Build history of the part. All positions in model axes, mm. A direction names the side the tool comes from. Coordinates: 2 decimals unless noted, no trailing zeros. Loops run counter-clockwise (first coordinate to the right, second up) from the corner with the lowest first, then second, coordinate; pieces in that order, holes last. Notation, with made-up numbers: (80, -6) - (100, -6) arc R29 cw to (100, 16) - close; hole circle Ø6 at (50, 14). An arc over 180 degrees is marked (long way). One line per item, written item: value.
```python
from build123d import *

# Parameters (mm, degrees)
F0_W      = 87.5036269426
F0_H      = 33.1910848618
F1_DEPTH  = 25.4
F1_FACE_W = 87.5036269426
F1_FACE_H = 33.1910848618
F2_DEPTH  = 9.3165077269
F2_TAPER  = -3


with BuildPart() as f1:
    # F0 (on Front) → F1 (new body)
    with BuildSketch(Plane.XZ):
        Rectangle(F0_W, F0_H)
    extrude(amount=F1_DEPTH)

    # F1_face (on face) → F2 (join)
    with BuildSketch(Plane.XZ.offset(25.4)):
        Rectangle(F1_FACE_W, F1_FACE_H)
    extrude(amount=-F2_DEPTH, taper=F2_TAPER)


solid = f1.part
```
Item 1: Drop flat-ended pins along their axis: P1, Ø8, axis at x = 7, y = -8.5, coming from the +Z side; P2, Ø5, axis at x = -5.5, y = -7.5, coming from the -Z side; P3, Ø5, axis at y = -4, z = 1, coming from the -X side. Give the stop position or say it passes through.
Check result:
P1: stops at z = 16.6
P2: stops at z = -16.6
P3: stops at x = -43.75
Item 2: Tool access for faces 1 (the face through (-1, -8, -16.596)), 2 (the face through (-1, -8, 16.596)), 3 (the face through (43.752, -8, 0)): list every direction of +Z, -Z, +X, -X, +Y, -Y with a clear straight run to the whole face (end or side of a thin tool).
Check result:
face 1: -Z, +X, -X, +Y
face 2: +Z, +X, -X, +Y
face 3: +Z, -Z, +X, +Y
Item 3: Probe probe 1 along X at (y, z) = (-7.5, 7); probe 2 along Z at (x, y) = (4, -1.75); probe 3 along X at (y, z) = (-19.25, 10.5). List the from-to ranges inside material, lowest first. Write a range as from..to.
Check result:
probe 1: x = -43.75..43.75
probe 2: z = -16.6..16.6
probe 3: x = -44.07..44.07
Item 4: Cut at A-A, the plane y = -1.75. Write the cut outline in (x, z), then the cut area to 3 significant figures.
Check result:
outline: (-43.75, -16.6) - (43.75, -16.6) - (43.75, 16.6) - (-43.75, 16.6) - close
area: 2,900 mm^2
